Design review of the part built by this model. Coordinates are the model's own, in mm. Coordinates: 2 decimals unless noted, no trailing zeros. Loops run counter-clockwise (first coordinate to the right, second up) from the corner with the lowest first, then second, coordinate; pieces in that order, holes last. Notation, with made-up numbers: (41.25, 50.25) -> (63.25, 50.25) arc R10 cw to (63.25, 62.25) -> close; hole circle Ø4 at (-10.5, 52.25). An arc over 180 degrees is marked (long way). Answer as a JSON object with one key per item and string values.
```python
from build123d import *

# Parameters (mm, degrees)
F1_DEPTH = 19
F2_R     = 5


with BuildPart() as f1:
    # F0 (on Top) → F1 (new body)
    with BuildSketch(Plane.XY):
        with BuildLine():
            Line((141.696946, 265.05909), (-101.57174, 265.05909))
            ThreePointArc((-101.57174, 265.05909), (-137.980527, 253.051325), (-160.102467, 221.73989))
            Line((-160.102467, 221.73989), (-160.102467, -66.769655))
            ThreePointArc((-160.102467, -66.769655), (-143.462282, -111.695054), (-101.57174, -134.94091))
            Line((-101.57174, -134.94091), (0, -134.94091))
            Line((0, -134.94091), (0, -245.450066))
            ThreePointArc((0, -245.450066), (25.285058, -270.735123), (50.570116, -245.450066))
            Line((50.570116, -245.450066), (50.570116, -134.94091))
            Line((50.570116, -134.94091), (141.409377, -134.94091))
            ThreePointArc((141.409377, -134.94091), (176.539135, -108.597939), (189.897533, -66.769655))
            Line((189.897533, -66.769655), (189.897533, 221.73989))
            ThreePointArc((189.897533, 221.73989), (174.100069, 252.637917), (141.696946, 265.05909))
        make_face()
    extrude(amount=F1_DEPTH)

    # F2
    f2_edges = [f1.edges().sort_by_distance(p)[0] for p in [
        (-160.102467, 221.73989, 9.5),
        (-160.102467, -66.769655, 9.5),
        (-160.102467, 77.485118, 0),
        (-160.102467, 77.485118, 19),
        (-101.57174, -134.94091, 9.5),
        (-143.462282, -111.695054, 0),
        (-143.462282, -111.695054, 19),
        (-50.78587, -134.94091, 19),
        (-50.78587, -134.94091, 0),
        (0, -134.94091, 9.5),
        (0, -245.450066, 9.5),
        (0, -190.195488, 0),
        (0, -190.195488, 19),
        (50.570116, -134.94091, 9.5),
        (141.409377, -134.94091, 9.5),
        (95.989746, -134.94091, 0),
        (95.989746, -134.94091, 19),
        (189.897533, -66.769655, 9.5),
        (176.539135, -108.597939, 0),
        (176.539135, -108.597939, 19),
        (189.897533, 221.73989, 9.5),
        (141.696946, 265.05909, 9.5),
        (174.100069, 252.637917, 0),
        (174.100069, 252.637917, 19),
    ]]
    fillet(f2_edges, radius=F2_R)


solid = f1.part
```
1) Add section C-C, the plane y = -177. Give the boundary of the cut face in (x, z), and give its area (3 significant figures).
Completed:
{"outline": "(0, 5) arc R5 ccw to (5, 0) -> (45.57, 0) arc R5 ccw to (50.57, 5) -> (50.57, 14) arc R5 ccw to (45.57, 19) -> (5, 19) arc R5 ccw to (0, 14) -> close", "area": "939 mm²"}
2) Add section A-A, the plane z = 8.25. Give the boundary of the cut face in (x, y), and give its area (3 significant figures).
Completed:
{"outline": "(-160.1, -66.77) arc R68.97 ccw to (-101.97, -134.88) arc R5 ccw to (-101.18, -134.94) -> (-5, -134.94) arc R5 cw to (0, -139.94) -> (0, -245.45) arc R25.29 ccw to (50.57, -245.45) -> (50.57, -139.94) arc R5 cw to (55.57, -134.94) -> (140.55, -134.94) arc R5 ccw to (142.25, -134.64) arc R72.17 ccw to (189.9, -66.77) -> (189.9, 221.47) arc R5 ccw to (189.87, 222.03) arc R48.48 ccw to (141.7, 265.06) -> (-101.57, 265.06) arc R61.2 ccw to (-159.86, 222.5) arc R5 ccw to (-160.1, 220.98) -> close", "area": "144,000 mm²"}
3) Wall thickness on probe 1 along Y at (x, z) = (-31.5, 7.25); probe 2 along X at (y, z) = (-180.5, 4.5); probe 3 along X at (y, z) = (-219, 9.25): over which ranges is each line inside the solid? List them lowest first.
Completed:
{"probe 1": "-134.94 to 265.06", "probe 2": "0.03 to 50.55", "probe 3": "0 to 50.57"}
4) Clearance check with flat-ended pins moving along their axes: pin 1 Ø10 at (x, z) = (-74, 9.5) entering from -Y; pin 2 Ø3 at (x, z) = (18.5, 4.5) entering from -Y; pin 3 Ø3 at (y, z) = (-160.5, 5.5) entering from +X. State where each tip first meets the part, or that it passes through.
Completed:
{"pin 1": "y = -134.94", "pin 2": "y = -270.17", "pin 3": "x = 50.57"}
5) Add section B-B, the plane x = 73. Give the boundary of the cut face in (y, z), and give its area (3 significant figures).
Completed:
{"outline": "(-134.94, 5) arc R5 ccw to (-129.94, 0) -> (260.06, 0) arc R5 ccw to (265.06, 5) -> (265.06, 14) arc R5 ccw to (260.06, 19) -> (-129.94, 19) arc R5 ccw to (-134.94, 14) -> close", "area": "7,580 mm²"}
